Input: part model. Units: mm. Frame: model coordinates. Coordinates: 2 decimals unless noted, no trailing zeros. Loops run counter-clockwise (first coordinate to the right, second up) from the corner with the lowest first, then second, coordinate; pieces in that order, holes last.
(1) Section B-B, the plane x = 0. Return loops of the section in (y, z), then the cut area to 3 significant figures.
(2) Line query: L1, parallel to Y at x = 1, z = 133.5; L2, parallel to X at y = 2.9, z = 202.5; L3, parallel to X at y = 2.8, z = 37. Output: solid intervals per line, ascending.
(3) Section A-A, the plane z = 86.5. Return loops of the section in (x, y), then the cut area to 3 significant figures.
(4) Mould query, pull axis X, two halves, no side actions, for faces 1 (the face through (0, 4.3, 158)), 2 (the face through (0, 3.229, 158)). Classes: released by +X, released by -X, zero draft, split by the parting line, or undercut.
(5) Contact query for a flat-ended pin moving along its axis: P1, Ø1.5, axis at x = 0, z = 166.5, coming from the -Y side. Output: stop coordinate, or through.
```python
from build123d import *

# Parameters (mm, degrees)
PAD_DEPTH = 320


with BuildPart() as part:
    # Sketch → Pad (new body)
    with BuildSketch(Plane.XY):
        with BuildLine():
            Line((-4.5, 4.3), (4.5, 4.3))
            Line((4.5, 4.3), (4.5, 4))
            Line((4.5, 4), (3.9, 4))
            Line((3.9, 4), (4.5, 2))
            Line((4.5, 2), (3.441966, 0))
            ThreePointArc((2.558034, 0.467615), (2.766192, -0.208159), (3.441966, 0))
            Line((2.558034, 0.467615), (3.368691, 2))
            Line((3.368691, 2), (3, 3.228972))
            Line((-3, 3.228972), (3, 3.228972))
            Line((-3, 3.228972), (-3.368691, 2))
            Line((-3.368691, 2), (-2.558034, 0.467615))
            ThreePointArc((-3.441966, 0), (-2.766192, -0.208159), (-2.558034, 0.467615))
            Line((-3.441966, 0), (-4.5, 2))
            Line((-4.5, 2), (-3.9, 4))
            Line((-3.9, 4), (-4.5, 4))
            Line((-4.5, 4), (-4.5, 4.3))
        make_face()
    extrude(amount=PAD_DEPTH)


solid = part.part
```
Report:
1. outline: (3.23, 0) - (4.3, 0) - (4.3, 320) - (3.23, 320) - close
1. area: 343 mm2
2. L1: y = 3.23 to 4.3
2. L2: x = -4.23 to -3.1, 3.1 to 4.23
2. L3: x = -4.26 to -3.13, 3.13 to 4.26
3. outline: (-4.5, 2) - (-3.44, 0) arc R0.5 ccw to (-2.56, 0.47) - (-3.37, 2) - (-3, 3.23) - (3, 3.23) - (3.37, 2) - (2.56, 0.47) arc R0.5 ccw to (3.44, 0) - (4.5, 2) - (3.9, 4) - (4.5, 4) - (4.5, 4.3) - (-4.5, 4.3) - (-4.5, 4) - (-3.9, 4) - close
3. area: 16.5 mm2
4. face 1: zero draft
4. face 2: undercut
5. P1: stops at y = 3.23
